Verification items for the finished model (mm, model axes). A direction names the side the tool comes from. Coordinates: 2 decimals unless noted, no trailing zeros. Order: outer loops, then holes, each group sorted by start corner. A loop starts at its lowest first (then second) coordinate and runs counter-clockwise, first axis right, second up.
Q1. Cross-section at C-C, the plane y = 80.5. Record the boundary of the cut face in (x, z).
Q2. Cross-section at A-A, the plane x = 0. Record the boundary of the cut face in (y, z), and give its area (3 significant figures).
Q3. Cross-section at D-D, the plane y = 14. Record the boundary of the cut face in (x, z).
Q4. Cross-section at B-B, the plane z = 0. Record the boundary of the cut face in (x, y), and give its area (3 significant figures).
Q5. Depth check by flat-ended pin: P1, Ø10, axis at x = 14.5, z = 2.5, coming from the +Y side; P2, Ø1, axis at y = 52, z = 4, coming from the -X side; P3, Ø6, axis at y = 9, z = 5, coming from the +X side; P4, Ø3, axis at y = 16.5, z = 1, coming from the +X side. Enter the tip coordinate at first touch or a pass-through.
Q6. Set-up check for faces 1 (the cylindrical face through (3.1, 52, 0.7)), 2 (the flat face through (0, 85.55, 0)): record each of +Z, -Z, +X, -X, +Y, -Y from which the full face is reachable in a straight line by a thin tool's end or side.
Q7. Thickness scan on line 1 (Y direction, x = 7.5, z = -12); line 2 (Y direction, x = 14.5, z = -12); line 3 (X direction, y = 44, z = 2). Record the ranges inside material, lowest first.
from build123d import *

# Parameters (mm, degrees)
FILLET1_R = 1.25


with BuildPart() as part:
    # Sketch1 → Revolve1 (revolve)
    with BuildSketch(Plane(origin=(0, 0, 0), x_dir=(0, 0, -1), z_dir=(1, 0, 0))):
        with BuildLine():
            Line((0, 0), (0, 85.55))
            Line((0, 85.55), (3.18, 85.55))
            Line((3.18, 85.55), (3.18, 20.623345081))
            ThreePointArc((3.18, 20.623345081), (8.570011584, 7.427407082), (22.50988431, 4.45))
            Line((22.50988431, 4.45), (26.67, 1.27))
            Line((26.67, 1.27), (26.67, 0))
            Line((26.67, 0), (0, 0))
        make_face()
    revolve(axis=Axis((0, 0, 0), (0, 1, 0)))

    # Fillet1
    fillet1_edges = [part.edges().sort_by_distance(p)[0] for p in [
        (0, 85.55, 3.18),
    ]]
    fillet(fillet1_edges, radius=FILLET1_R)


solid = part.part
Check values:
1. outline: circle Ø6.36 at (0, 0)
2. outline: (0, -26.67) - (1.27, -26.67) - (4.45, -22.51) arc R15.25 cw to (20.62, -3.18) - (84.3, -3.18) arc R1.25 ccw to (85.55, -1.93) - (85.55, 1.93) arc R1.25 ccw to (84.3, 3.18) - (20.62, 3.18) arc R15.25 cw to (4.45, 22.51) - (1.27, 26.67) - (0, 26.67) - close
2. area: 816 mm2
3. outline: circle Ø7.98 at (0, 0)
4. outline: (-26.67, 0) - (26.67, 0) - (26.67, 1.27) - (22.51, 4.45) arc R15.25 cw to (3.18, 20.62) - (3.18, 84.3) arc R1.25 ccw to (1.93, 85.55) - (-1.93, 85.55) arc R1.25 ccw to (-3.18, 84.3) - (-3.18, 20.62) arc R15.25 cw to (-22.51, 4.45) - (-26.67, 1.27) - close
4. area: 816 mm2
5. P1: stops at y = 6.56
5. P2: passes through
5. P3: stops at x = 9.52
5. P4: stops at x = 3.62
6. face 1: +Y
6. face 2: +Z, -Z, +X, -X, +Y
7. line 1: y = 0 to 4.46
7. line 2: y = 0 to 3.88
7. line 3: x = -2.47 to 2.47
